Geometry: final body of the model. Coordinates: model frame, mm. A direction names the side the tool comes from. Round coordinates to 2 decimals unless told otherwise and drop trailing zeros. Loops run counter-clockwise (first coordinate to the right, second up) from the corner with the lowest first, then second, coordinate; pieces in that order, holes last. Notation, with made-up numbers: (-16, 9.25) - (-2, 9.25) arc R30 ccw to (-2, 48.25) - close; hole circle Ø8 at (-35, 56). An arc over 180 degrees is marked (long way). Return JSON: item names as keys, results as strings. Group by question number.
1. Section D-D on z = 560.5. Return loops of the section in (x, y).
2. Section A-A on z = 641.64. Return loops of the section in (x, y), and give its area (3 significant figures).
3. First-contact query: pin 1 Ø7 at (x, y) = (-12.5, 28.5) entering from +Z; pin 2 Ø15 at (y, z) = (-4.5, 702.5) entering from -X; pin 3 Ø1.5 at (y, z) = (-28, 582) entering from +X; pin 4 Ø20 at (x, z) = (0, 721.64) entering from -Y. Flat tips, straight axial feed; report the tip coordinate or a pass-through.
4. Section C-C on x = -45.5. Return loops of the section in (y, z), and give its area (3 significant figures).
5. Draft query along Y for faces 1 (the face through (34.369, 0, 704)), 2 (the face through (0, 15, 705)), 3 (the face through (0, 0, 664)). Return one class per face: +Y half, -Y half, draft (parallel to the pull), parting line (faces both ways), or undercut.
6. Set-up query: faces 4 (the face through (-63.95, 6.76, 663.1)), 5 (the face through (0, 24, 686)), 6 (the face through (-34.369, 0, 704)), 7 (the face through (0, -24, 686)). Return all of +Z, -Z, +X, -X, +Y, -Y with unobstructed straight access to the full face (end or side cutting, diameter ignored); none if empty.
7. Material intervals for probe 1 along Y at (x, z) = (1.5, 267); probe 2 along Y at (x, z) = (0, 146.5); probe 3 along Z at (x, y) = (0, -6.5), sorted ascending.
from build123d import *

# Parameters (mm, degrees)
SKETCH1_R           = 37.5
SKETCH1_R_2         = 17.5
BOSS_EXTRUDE1_DEPTH = 664
SKETCH5_R           = 37.5
BOSS_EXTRUDE2_DEPTH = 22
SKETCH8_W           = 68.738635424
SKETCH8_H           = 15
BOSS_EXTRUDE3_DEPTH = 70
FILLET1_R           = 34.36
SKETCH9_R           = 12.5
CUT_EXTRUDE1_DEPTH  = 100
SKETCH10_R          = 22.5
BOSS_EXTRUDE4_DEPTH = 60


with BuildPart() as part:
    # Sketch1 → Boss-Extrude1 (new body)
    with BuildSketch(Plane.XY):
        Circle(SKETCH1_R)
        Circle(SKETCH1_R_2, mode=Mode.SUBTRACT)
    extrude(amount=BOSS_EXTRUDE1_DEPTH)

    # Sketch5 → Boss-Extrude2 (add)
    with BuildSketch(Plane.XY.offset(664)):
        Circle(SKETCH5_R)
    extrude(amount=BOSS_EXTRUDE2_DEPTH)

    # Sketch8 → Boss-Extrude3 (add)
    with BuildSketch(Plane.XY.offset(686)):
        with Locations((0, -7.5)):
            Rectangle(SKETCH8_W, SKETCH8_H)
    boss_extrude3 = extrude(amount=BOSS_EXTRUDE3_DEPTH)

    # Mirror1: Boss-Extrude3 across plane
    add(boss_extrude3.mirror(Plane(origin=(-34.369317712, 0, 756), x_dir=(0, 0, 1), z_dir=(0, -1, 0))))

    # Fillet1
    fillet1_edges = [part.edges().sort_by_distance(p)[0] for p in [
        (-34.369317712, 0, 756),
        (34.369317712, 0, 756),
    ]]
    fillet(fillet1_edges, radius=FILLET1_R)

    # Sketch9 → Cut-Extrude1 (cut, symmetric)
    with BuildSketch(Plane(origin=(0, 15, 0), x_dir=(1, 0, 0), z_dir=(0, 1, 0))):
        with Locations((0, -721.64)):
            Circle(SKETCH9_R)
    extrude(amount=CUT_EXTRUDE1_DEPTH, both=True, mode=Mode.SUBTRACT)

    # Sketch10 → Boss-Extrude4 (add)
    with BuildSketch(Plane.ZY.offset(34.369317712)):
        with Locations((641.64, 0)):
            Circle(SKETCH10_R)
    extrude(amount=BOSS_EXTRUDE4_DEPTH)


solid = part.part
Taken from the geometry:
{
 "1": {"outline": "circle Ø75 at (0, 0); hole circle Ø35 at (0, 0)"},
 "2": {"outline": "(-94.37, -22.5) - (-34.37, -22.5) - (-34.37, -15) arc R37.5 ccw (long way) to (-34.37, 15) - (-34.37, 22.5) - (-94.37, 22.5) - close; hole circle Ø35 at (0, 0)", "area": "6,090 mm2"},
 "3": {"pin 1": "z = 686", "pin 2": "x = -34.37", "pin 3": "x = 25.76", "pin 4": "through"},
 "4": {"outline": "circle Ø45 at (0, 641.64)", "area": "1,590 mm2"},
 "5": {"face 1": "draft", "face 2": "+Y half", "face 3": "undercut"},
 "6": {"face 4": "-X", "face 5": "+Z, +X, -X, +Y", "face 6": "+Z, -X, +Y, -Y", "face 7": "+Z, +X, -X, -Y"},
 "7": {"probe 1": "-37.47 to -17.44, 17.44 to 37.47", "probe 2": "-37.5 to -17.5, 17.5 to 37.5", "probe 3": "664 to 709.14, 734.14 to 756"}
}
